Verification items for this drawing (mm, ordinates from the low corner). A direction names the side the tool comes from. Give positions to 0.01 mm unless a question says otherwise; leave off trailing zeros. Write each loop counter-clockwise with the first axis right and the second up, starting at its lowest first coordinate (ties: lowest second). Pieces come first, ordered by that corner, then holes. Notation, with made-up numbers: M -14,89.25 L 44,89.25 A29 cw 44,116.25 Z; hole C 1,66.5 d5. An arc over 180 degrees is marked long. Write each question's results on one line, items separated by ' | '.
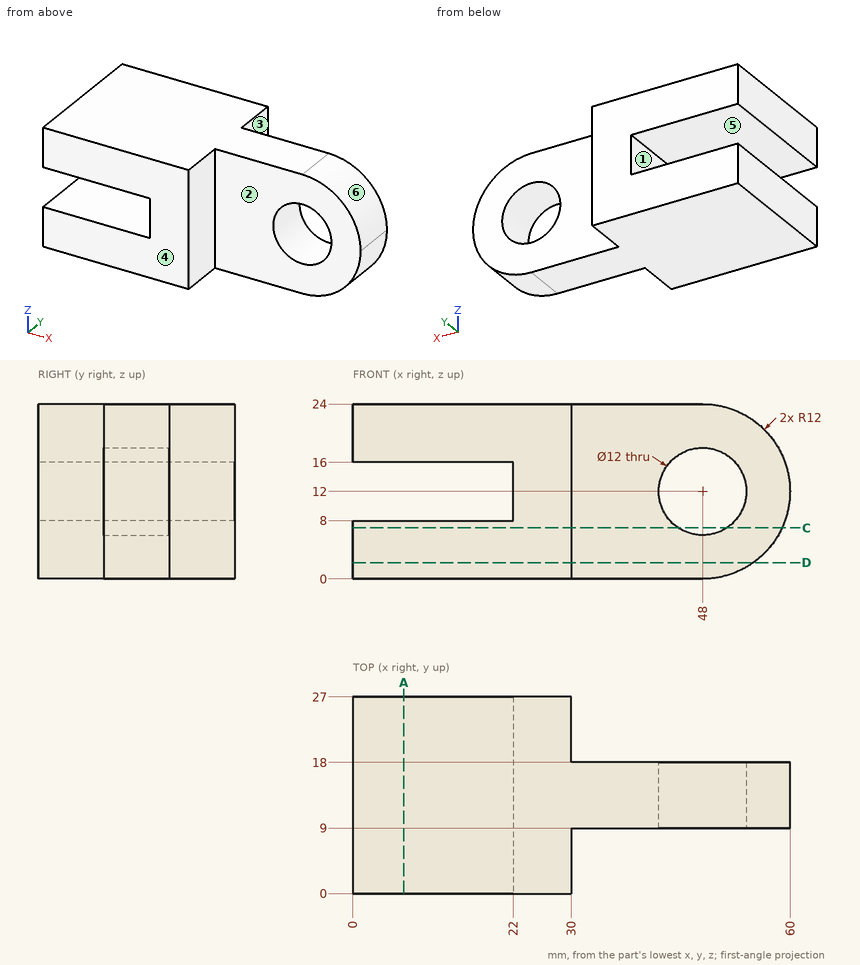
Q1. Release check for a two-part mould opening along Z. For the marked faces 4, 5 and 6 record: released by +Z, released by -Z, zero draft, split by the parting line, or undercut.
Answer key:
face 4: zero draft | face 5: undercut | face 6: released by +Z
Q2. Section check D-D (z = 2.25). Enter the section's corners in (x, y), then the cut area to 3 significant figures.
Answer key:
outline: M 0,0 L 30,0 L 30,9 L 55,9 L 55,18 L 30,18 L 30,27 L 0,27 Z | area: 1,030 mm2
Q3. Section check A-A (x = 7). Enter the section's corners in (y, z).
Answer key:
outline: M 0,0 L 27,0 L 27,8 L 0,8 Z; M 0,16 L 27,16 L 27,24 L 0,24 Z
Q4. Depth check by flat-ended pin: P1, Ø8, axis at x = 53, z = 16.5, coming from the +Y side; P2, Ø10, axis at x = 33.5, y = 10.5, coming from the -Z side; P3, Ø2.5, axis at y = 24.5, z = 17, coming from the +X side. Enter the tip coordinate at first touch or a pass-through.
Answer key:
P1: stops at y = 18 | P2: stops at z = 0 | P3: stops at x = 30
Q5. Access from +Z, -Z, +X, -X, +Y, -Y to the whole of each face (thin tool, end or side, straight path). Record for the marked faces 1, 2 and 3.
Answer key:
face 1: -X, +Y, -Y | face 2: +Z, -Z, +X, -Y | face 3: +Z, -Z, +X, +Y
Q6. Material ranges on probe 1 along X at (y, z) = (16, 12); probe 2 along Z at (x, y) = (48, 12.75); probe 3 along Z at (x, y) = (15, 15.25), recorded low to high. Write a range as [from, to].
Answer key:
probe 1: x = [22, 42], [54, 60] | probe 2: z = [0, 6], [18, 24] | probe 3: z = [0, 8], [16, 24]
Q7. Section check C-C (z = 7). Enter the section's corners in (x, y).
Answer key:
outline: M 0,0 L 30,0 L 30,9 L 44.68,9 L 44.68,18 L 30,18 L 30,27 L 0,27 Z; M 51.32,9 L 58.91,9 L 58.91,18 L 51.32,18 Z
